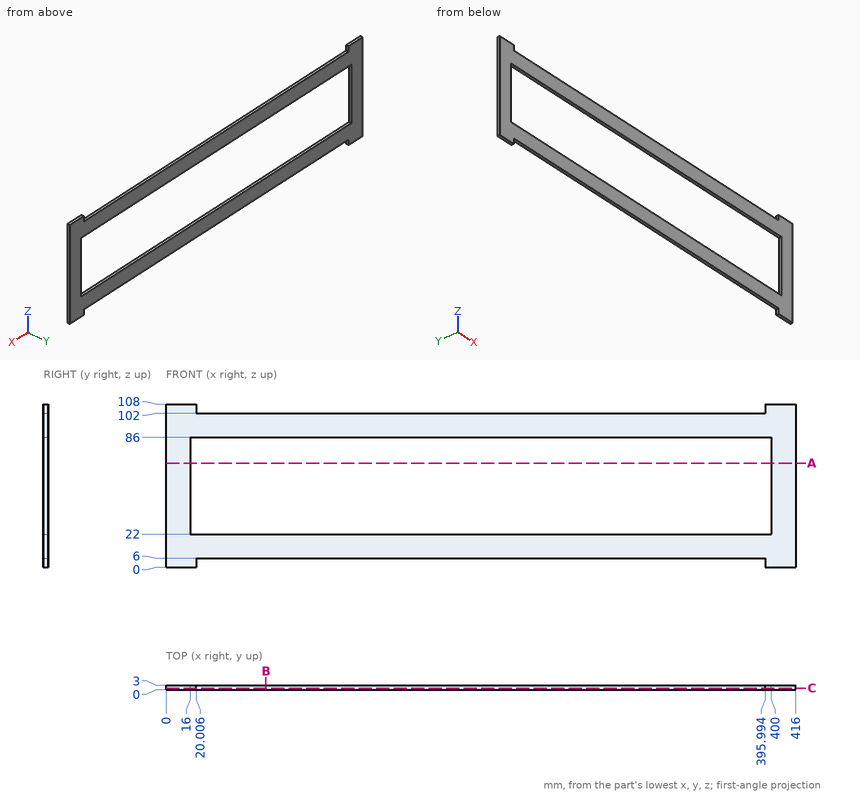
Input: dimensioned drawing with shaded views. Units: mm. Origin: part minimum x, y, z. Round coordinates to 2 decimals unless told otherwise and drop trailing zeros. Loops run counter-clockwise (first coordinate to the right, second up) from the corner with the lowest first, then second, coordinate; pieces in that order, holes last. Notation, with made-up numbers: M -6,23 L 19,23 A25 cw 19,59 Z; hole C -39,70 d1. An arc over 180 degrees is marked long. Answer in a Markdown table with one row per item. Add a question column.
1. Contact query for flat-ended pins moving along their axis: pin 1 (1.5 mm diameter, centred on x = 139.5, y = 1.5, fed in from +Z); pin 2 (0.9 mm diameter, centred on x = 248.5, y = 1.5, fed in from -Z). Output: stop coordinate, or through.
2. Ray query, probe 1 along Z at (x, y) = (98.5, 1.5); probe 2 along X at (y, z) = (2.15, 30.5). Return the intervals inside material, ascending.
3. Section B-B (x = 66). Output: boundary loops of the cut face in (y, z).
4. Section A-A (z = 69). Output: boundary loops of the cut face in (x, y), and give its area (3 significant figures).
5. Section C-C (y = 1.15). Output: boundary loops of the cut face in (x, z).
Values follow:
| question | item | result |
|---|---|---|
| 1 | pin 1 | z = 102 |
| 1 | pin 2 | z = 6 |
| 2 | probe 1 | 6 to 22, 86 to 102 |
| 2 | probe 2 | 0 to 16, 400 to 416 |
| 3 | outline | M 0,6 L 3,6 L 3,22 L 0,22 Z; M 0,86 L 3,86 L 3,102 L 0,102 Z |
| 4 | outline | M 0,0 L 16,0 L 16,3 L 0,3 Z; M 400,0 L 416,0 L 416,3 L 400,3 Z |
| 4 | area | 96.0 mm^2 |
| 5 | outline | M 0,0 L 20.01,0 L 20.01,6 L 395.99,6 L 395.99,0 L 416,0 L 416,108 L 395.99,108 L 395.99,102 L 20.01,102 L 20.01,108 L 0,108 Z; hole M 16,22 L 400,22 L 400,86 L 16,86 Z |
